from build123d import *

# Parameters (mm, degrees)
SKETCH1_W           = 15.875
SKETCH1_H           = 7.9375
BOSS_EXTRUDE1_DEPTH = 9.525
SKETCH2_R           = 2.38125
BOSS_EXTRUDE2_DEPTH = 1.5875
LPATTERN1_COUNT     = 2
LPATTERN1_PITCH     = 7.9375
SHELL3_T            = -1.5875
SKETCH3_R           = 1.5875
BOSS_EXTRUDE3_DEPTH = 7.9375


with BuildPart() as part:
    # Sketch1 → Boss-Extrude1 (new body)
    with BuildSketch(Plane.XY):
        with Locations((7.9375, 3.96875)):
            Rectangle(SKETCH1_W, SKETCH1_H)
    extrude(amount=BOSS_EXTRUDE1_DEPTH)

    # Sketch2 → Boss-Extrude2 (add)
    with BuildSketch(Plane.XY.offset(9.525)):
        with Locations((3.96875, 3.96875)):
            Circle(SKETCH2_R)
    boss_extrude2 = extrude(amount=BOSS_EXTRUDE2_DEPTH)

    # LPattern1: Boss-Extrude2 ×2
    with Locations(*[(i * LPATTERN1_PITCH, 0, 0) for i in range(1, LPATTERN1_COUNT)]):
        add(boss_extrude2)

    # Shell3
    shell3_openings = [part.faces().sort_by_distance(p)[0] for p in [
        (7.9375, 3.96875, 0),
    ]]
    offset(amount=SHELL3_T, openings=shell3_openings, kind=Kind.INTERSECTION)

    # Sketch3 → Boss-Extrude3 (add)
    with BuildSketch(Plane(origin=(0, 0, 7.9375), x_dir=(-1, 0, 0), z_dir=(0, 0, -1))):
        with Locations((-7.9375, 3.96875)):
            Circle(SKETCH3_R)
    extrude(amount=BOSS_EXTRUDE3_DEPTH)


solid = part.part
Build history of the part. All positions in model axes, mm. A direction names the side the tool comes from. Round coordinates to 2 decimals unless told otherwise and drop trailing zeros. Write each loop counter-clockwise with the first axis right and the second up, starting at its lowest first coordinate (ties: lowest second). Pieces come first, ordered by that corner, then holes. Notation, with made-up numbers: M -26.75,10.25 L -13.75,10.25 A30 cw -13.75,39.25 Z; hole C 85.5,34 d4. An arc over 180 degrees is marked long. Answer in a Markdown table with one row per item.
1. Saw through at A-A (z = 4.5). State how many separate pieces and enclosed holes the cut face has, and give its area (3 significant figures).
Geometry check:
| item | result |
|---|---|
| separate pieces | 2 |
| enclosed holes | 1 |
| area | 73.4 mm2 |
2. Saw through at D-D (z = 9). List the corners of the cut face in (x, y) (1 decimal).
Geometry check:
| item | result |
|---|---|
| outline | M 0,0 L 15.9,0 L 15.9,7.9 L 0,7.9 Z; hole C 4,4 d1.6; hole C 11.9,4 d1.6 |
3. Mould opens along Y. For faces 1 (the face through (8, 0, 5)), 2 (the face through (15.875, 4, 5)), 3 (the face through (8, 7.938, 5)), 4 (the face through (8, 6.35, 4)) say: +Y half, -Y half, draft (parallel to the pull), parting line (faces both ways), or undercut.
Geometry check:
| item | result |
|---|---|
| face 1 | -Y half |
| face 2 | draft |
| face 3 | +Y half |
| face 4 | undercut |
4. Flat gauge pins, fed straight in: P1, Ø1, axis at y = 7, z = 4.5, coming from the -X side; P2, Ø0.5, axis at x = 4, y = 4, coming from the -Z side (3 decimals). Where does each tip first touch, or does it go through?
Geometry check:
| item | result |
|---|---|
| P1 | x = 0 |
| P2 | z = 9.525 |
5. Saw through at C-C (y = 4.5). List the corners of the cut face in (x, z) (1 decimal), and give its area (3 significant figures).
Geometry check:
| item | result |
|---|---|
| outline | M 0,0 L 1.6,0 L 1.6,7.9 L 3.4,7.9 L 3.4,9.5 L 4.6,9.5 L 4.6,7.9 L 6.4,7.9 L 6.4,0 L 9.4,0 L 9.4,7.9 L 11.3,7.9 L 11.3,9.5 L 12.5,9.5 L 12.5,7.9 L 14.3,7.9 L 14.3,0 L 15.9,0 L 15.9,9.5 L 14.2,9.5 L 14.2,11.1 L 9.6,11.1 L 9.6,9.5 L 6.3,9.5 L 6.3,11.1 L 1.6,11.1 L 1.6,9.5 L 0,9.5 Z |
| area | 85.1 mm2 |
6. Which spindle directions (+Z, -Z, +X, -X, +Y, -Y) get a long thin tool onto all of the face, cutting with end or side? Do faces 5 (the face through (10.151, 5.578, 10.308)), 6 (the face through (6, 5, 7.938)), 7 (the face through (12, 4, 11.112)). Say none if no direction does.
Geometry check:
| item | result |
|---|---|
| face 5 | +Z |
| face 6 | -Z |
| face 7 | +Z, +X, -X, +Y, -Y |
7. Probe L1, parallel to X at y = 4, z = 4.5 (1 decimal); L2, parallel to Y at x = 8, z = 3.75; L3, parallel to X at y = 1.75, z = 5.75 (1 decimal). List the from-to ranges inside material, lowest first. Write a range as [from, to].
Geometry check:
| item | result |
|---|---|
| L1 | [0, 1.6], [6.4, 9.5], [14.3, 15.9] |
| L2 | [0, 1.59], [2.38, 5.56], [6.35, 7.94] |
| L3 | [0, 1.6], [14.3, 15.9] |
